Geometry check sheet. Reference: the model listing, model coordinates, mm. A direction names the side the tool comes from. Round coordinates to 2 decimals unless told otherwise and drop trailing zeros. Loops run counter-clockwise (first coordinate to the right, second up) from the corner with the lowest first, then second, coordinate; pieces in that order, holes last. Notation, with made-up numbers: M 22,-31.75 L 39,-31.75 A17 ccw 39,-10.75 Z; hole C 19.25,-19.75 d9. An arc over 180 degrees is marked long. Use one line per item in the form item = value. Start each with the question number.
1. Cross-section at B-B (z = 11.4). Record the boundary of the cut face in (x, y) (3 decimals), then the cut area to 3 significant figures.
2. Cross-section at D-D (z = 3.6). Record the boundary of the cut face in (x, y) (3 decimals), then the cut area to 3 significant figures.
3. Cross-section at A-A (x = 3.75). Record the boundary of the cut face in (y, z), then the cut area to 3 significant figures.
4. Cross-section at C-C (y = 19.5). Record the boundary of the cut face in (x, z) (3 decimals), then the cut area to 3 significant figures.
5. Go/stop test with flat-tipped pins: pin 1 (5 mm diameter, centred on y = 12, z = 13, fed in from -X); pin 2 (1.5 mm diameter, centred on y = 9, z = 9, fed in from +X); pin 3 (2 mm diameter, centred on y = 8, z = 10, fed in from +X); pin 4 (2.5 mm diameter, centred on y = 14.5, z = 5, fed in from -X). Record where each tip stops, or that it passes through.
6. Set-up check for faces 1 (the flat face through (3, 11, 7.2)), 2 (the flat face through (-6.36, 13.92, 14.49)), 3 (the flat face through (-10, 20.2, 14.5)): record each of +Z, -Z, +X, -X, +Y, -Y from which the full face is reachable in a straight line by a thin tool's end or side.
7. Material ranges on line 1 (Z direction, x = 3.75, y = 6.5); line 2 (Z direction, x = -4.25, y = 2.5); line 3 (Y direction, x = -13.75, z = 7), recorded low to high.
8. Draft check along Z on faces 4 (the cylindrical face through (-4.41, 11.03, 9.98)), 5 (the flat face through (-10.1, 19.7, 0.6)), 6 (the flat face through (-9, 17.65, 7)). Enter one of: pulls with the +Z half, pulls with the -Z half, needs draft (parallel to the pull), parting line crosses it, or undercut.
```python
from build123d import *

# Parameters (mm, degrees)
RESSALTO_EXTRUS_O1_DEPTH = 15
CORTE_EXTRUS_O1_REACH    = 32.259
ESBO_O2_R                = 1.6
ESBO_O3_W                = 7.5
ESBO_O3_H                = 7.2
ESBO_O3_R                = 1.6
RESSALTO_EXTRUS_O2_DEPTH = 21.75
FILETE1_R                = 2
FILETE2_R                = 3
CHANFRO1_SIZE            = 1
CHANFRO2_SIZE            = 1


with BuildPart() as part:
    # Esboço1 → Ressalto-extrusão1 (new body)
    with BuildSketch(Plane.XY):
        Polygon((0, 0), (0, 21.75), (-10.5, 21.75), (-10.5, 17.65), (-6.85, 17.65), (-6.85, 10.05), (-14.75, 10.05), (-14.75, 0), align=None)
    extrude(amount=RESSALTO_EXTRUS_O1_DEPTH)

    # Esboço2 → Corte-extrusão1 (cut, up to next)
    with BuildSketch(Plane(origin=(0, 21.75, 0), x_dir=(1, 0, 0), z_dir=(0, 1, 0)), mode=Mode.PRIVATE) as corte_extrus_o1_sk1:
        with Locations(Location((-3.675, -3.6, 0), (0, 0, 180))):
            Circle(ESBO_O2_R)
    corte_extrus_o1_tool1 = extrude(corte_extrus_o1_sk1.sketch, amount=-CORTE_EXTRUS_O1_REACH, mode=Mode.PRIVATE) & part.part
    # Esboço2 → Corte-extrusão1 (cut, up to next)
    with BuildSketch(Plane(origin=(0, 21.75, 0), x_dir=(1, 0, 0), z_dir=(0, 1, 0)), mode=Mode.PRIVATE) as corte_extrus_o1_sk2:
        with Locations(Location((-3.675, -11.4, 0), (0, 0, 180))):
            Circle(ESBO_O2_R)
    corte_extrus_o1_tool2 = extrude(corte_extrus_o1_sk2.sketch, amount=-CORTE_EXTRUS_O1_REACH, mode=Mode.PRIVATE) & part.part
    add(corte_extrus_o1_tool1.solids().sort_by_distance((-3.675, 21.75, 3.6))[0], mode=Mode.SUBTRACT)
    add(corte_extrus_o1_tool2.solids().sort_by_distance((-3.675, 21.75, 11.4))[0], mode=Mode.SUBTRACT)

    # Esboço3 → Ressalto-extrusão2 (add)
    with BuildSketch(Plane(origin=(0, 21.75, 0), x_dir=(1, 0, 0), z_dir=(0, 1, 0))):
        with Locations((3.75, -3.6)):
            Rectangle(ESBO_O3_W, ESBO_O3_H)
        with Locations(Location((3.75, -3.6, 0), (0, 0, 180))):
            Circle(ESBO_O3_R, mode=Mode.SUBTRACT)
    extrude(amount=-RESSALTO_EXTRUS_O2_DEPTH)

    # Filete1
    filete1_edges = [part.edges().sort_by_distance(p)[0] for p in [
        (0, 10.875, 7.2),
    ]]
    fillet(filete1_edges, radius=FILETE1_R)

    # Filete2
    filete2_edges = [part.edges().sort_by_distance(p)[0] for p in [
        (7.5, 10.875, 7.2),
        (0, 10.875, 15),
    ]]
    fillet(filete2_edges, radius=FILETE2_R)

    # Chanfro1
    chanfro1_edges = [part.edges().sort_by_distance(p)[0] for p in [
        (-3.625, 0, 0),
        (7.5, 10.875, 0),
        (-14.75, 5.025, 0),
        (-10.8, 10.05, 0),
        (-6.85, 13.85, 0),
        (-8.675, 17.65, 0),
        (-10.5, 19.7, 0),
        (-1.5, 21.75, 0),
    ]]
    chamfer(chanfro1_edges, length=CHANFRO1_SIZE)

    # Chanfro2
    chanfro2_edges = [part.edges().sort_by_distance(p)[0] for p in [
        (-10.5, 19.7, 15),
        (-8.675, 17.65, 15),
        (-6.85, 13.85, 15),
        (-10.8, 10.05, 15),
        (-14.75, 5.025, 15),
    ]]
    chamfer(chanfro2_edges, length=CHANFRO2_SIZE)


solid = part.part
```
Reported:
q1.outline = M -14.75,0 L -5.275,0 L -5.275,21.75 L -10.5,21.75 L -10.5,17.65 L -6.85,17.65 L -6.85,10.05 L -14.75,10.05 Z; M -2.075,0 L 0,0 L 0,21.75 L -2.075,21.75 Z
q1.area = 174 mm²
q2.outline = M -14.75,0 L -5.275,0 L -5.275,21.75 L -10.5,21.75 L -10.5,17.65 L -6.85,17.65 L -6.85,10.05 L -14.75,10.05 Z; M -2.075,0 L 2.15,0 L 2.15,21.75 L -2.075,21.75 Z; M 5.35,0 L 7.5,0 L 7.5,21.75 L 5.35,21.75 Z
q2.area = 267 mm²
q3.outline = M 0,1 L 1,0 L 20.75,0 L 21.75,1 L 21.75,2 L 0,2 Z; M 0,5.2 L 21.75,5.2 L 21.75,7.2 L 0,7.2 Z
q3.area = 86.0 mm²
q4.outline = M -10.5,1 L -9.5,0 L 6.5,0 L 7.5,1 L 7.5,4.2 A3 ccw 4.5,7.2 L 2,7.2 A2 cw 0,9.2 L 0,12 A3 ccw -3,15 L -9.5,15 L -10.5,14 Z; hole C -3.675,3.6 d3.2; hole C -3.675,11.4 d3.2; hole C 3.75,3.6 d3.2
q4.area = 183 mm²
q5.pin_1 = -14.75
q5.pin_2 = 0.24
q5.pin_3 = 0.01
q5.pin_4 = -6.85
q6.face_1 = +Z, +X, +Y, -Y
q6.face_2 = +Z, -X
q6.face_3 = +Z, -X, +Y
q7.line_1 = 0 to 2, 5.2 to 7.2
q7.line_2 = 0 to 2.11, 5.09 to 9.91, 12.89 to 15
q7.line_3 = 0 to 10.05
q8.face_4 = undercut
q8.face_5 = pulls with the -Z half
q8.face_6 = needs draft
